Autodesk Inventor part; units mm, degrees
ref_plane "YZ Plane" through (0, 0, 0) normal (1, 0, 0) x (0, 1, 0)
ref_plane "XZ Plane" through (0, 0, 0) normal (0, 1, 0) x (-1, 0, 0)
ref_plane "XY Plane" through (0, 0, 0) normal (0, 0, 1) x (1, 0, 0)
sketch "Sketch1" plane through (0, 0, 0) normal (0, 1, 0) x (-1, 0, 0)
  circle A0 centre (0, 0) radius 3.5
  circle A1 centre (0, 0) radius 3.9
  circle A2 centre (0, 0) radius 0.5
  line L0 (3.9, 0) -> (3.9, 3.9)
  line L1 (3.9, 3.9) -> (0, 3.9)
  line L2 (-3.9, 0) -> (-3.9, 3.9)
  line L3 (-3.9, 3.9) -> (0, 3.9)
  line L4 (3.9, 3.9) -> (3.9, 5.9)
  line L5 (3.9, 5.9) -> (-3.9, 5.9)
  line L6 (-3.9, 5.9) -> (-3.9, 3.9)
  line L7 (3.9, 5.9) -> (10, 5.9)
  line L8 (10, 5.9) -> (10, 3.9)
  line L9 (10, 3.9) -> (3.9, 3.9)
  line L10 (-3.9, 5.9) -> (-10, 5.9)
  line L11 (-10, 5.9) -> (-10, 3.9)
  line L12 (-10, 3.9) -> (-3.9, 3.9)
  dimension "d0" = 7
  dimension "d1" = 7.8
  dimension "d2" = 1
  dimension "d7" = 2
  dimension "d10" = 20
extrude "Extrusion1" add sketch "Sketch1" along normal blind 8 contours A1 | A1 L1 L0 | L3 L6 L5 L4 L1 | A1 L2 L3 | L4 L7 L8 L9 | L12 L11 L10 L6
extrude "Extrusion2" add sketch "Sketch1" against normal blind 2 contours A0 | A1 | A1 L1 L0 | L3 L6 L5 L4 L1 | A1 L2 L3 | L4 L7 L8 L9 | L12 L11 L10 L6
sketch "Sketch2" plane through (10, 8, 3.9) normal (0, 0, -1) x (-1, 0, 0)
  circle A0 centre (3, -5) radius 1.5
  circle A1 centre (17, -5) radius 1.5
  line L0 (3, -5) -> (17, -5) construction
  line L1 (0, -10) -> (0, 0) construction
  line L2 (20, -10) -> (20, 0) construction
  line L3 (0, 0) -> (6.1, 0)
  line L4 (3, -3.5) -> (3, -3) construction
  line L5 (3, -3) -> (3.9922, -3.875)
  line L6 (3, -3) -> (2.0078, -3.875)
  line L7 (17, -3.5) -> (17, -3) construction
  line L8 (17, -3) -> (16.0078, -3.875)
  line L9 (17, -3) -> (17.9922, -3.875)
  point P0 (10, -8)
  dimension "d11" = 3
  dimension "d12" = 3
  dimension "d13" = 3
  dimension "d14" = 3
  dimension "d15" = 5
  dimension "d18" = 0.5
  dimension "d19" = 0.5
extrude "Extrusion3" cut sketch "Sketch2" against normal through all
equation "\"d13\" = d12"
equation "\"d14\" = d11"
equation "\"d19\" = d18"
properties part number "w_3DPrint"
Here's how the part is built. I have some questions about the finished solid (model axes, mm). A direction names the side the tool comes from. Give positions to 0.01 mm unless a question says otherwise; leave off trailing zeros. Order: outer loops, then holes, each group sorted by start corner. A loop starts at its lowest first (then second) coordinate and runs counter-clockwise, first axis right, second up. Notation, with made-up numbers: (39.5, -20.5) -> (78.5, -20.5) arc R32 ccw to (78.5, 5.5) -> close; hole circle Ø10 at (79, -30.5). An arc over 180 degrees is marked (long way). Use a Markdown table: item, result. Add a question column.
Item 1: Will these pins go through, and if not, where does the flat tip stop? pin 1 (1.2 mm diameter, centred on y = 2.5, z = 2, fed in from -X); pin 2 (2 mm diameter, centred on x = 6, y = 5.5, fed in from -Z); pin 3 (3.5 mm diameter, centred on x = 0.5, z = 1, fed in from +Y).
Item 2: Imagine slicing it at A-A on y = 3. Please give me the cut outline in (x, z).
Item 3: I need wall thicknesses on line 1 (X direction, y = 3, z = 4.95); line 2 (Z direction, x = 0, y = -0.85); line 3 (Z direction, x = -5, y = 7.5). Which ranges of each line are inside material? Lowest first, please.
Item 4: For faces 1 (the face through (-8.3, 1.8, 3.9)), 2 (the face through (3.9, 3, 2)), 3 (the face through (-3.233, 3.944, 1.341)), 4 (the face through (-7.49, 4.57, 4.89)), which set-ups out of +Z, -Z, +X, -X, +Y, -Y let a thin tool reach every point of the face, with its end or its side?
Item 5: If we mould it in two halves opening along Y, with no side actions, what happens to faces 5 (the face through (0, 0, -1)), 6 (the face through (7.49, 4.57, 4.89)), 7 (the face through (10, 3, 5))? For each: pulls with the +Y half, pulls with the -Y half, needs draft (parallel to the pull), parting line crosses it, or undercut.
Item 6: Imagine slicing it at D-D on z = -1. Please give me the cut outline in (x, y), plus the area to 3 significant figures.
Item 7: Imagine slicing it at B-B on x = 6.5. Please give me the cut outline in (y, z).
Item 8: Imagine slicing it at C-C on y = -0.75. Please give me the cut outline in (x, z).
Data:
| question | item | result |
|---|---|---|
| 1 | pin 1 | stops at x = -3.9 |
| 1 | pin 2 | stops at z = 3.9 |
| 1 | pin 3 | stops at y = 0 |
| 2 | outline | (-10, 3.9) -> (-8.5, 3.9) -> (-8.5, 5.9) -> (-10, 5.9) -> close; (-5.5, 3.9) -> (-3.9, 3.9) -> (-3.9, 0) arc R3.9 ccw to (3.9, 0) -> (3.9, 3.9) -> (5.5, 3.9) -> (5.5, 5.9) -> (-5.5, 5.9) -> close; (8.5, 3.9) -> (10, 3.9) -> (10, 5.9) -> (8.5, 5.9) -> close; hole circle Ø7 at (0, 0) |
| 3 | line 1 | x = -10 to -8.5, -5.5 to 5.5, 8.5 to 10 |
| 3 | line 2 | z = -3.9 to -0.5, 0.5 to 5.9 |
| 3 | line 3 | z = 3.9 to 5.9 |
| 4 | face 1 | -Z, -X, +Y, -Y |
| 4 | face 2 | -Z, +X, +Y, -Y |
| 4 | face 3 | +Y |
| 4 | face 4 | +Z, -Z |
| 5 | face 5 | pulls with the +Y half |
| 5 | face 6 | undercut |
| 5 | face 7 | needs draft |
| 6 | outline | (-3.77, -2) -> (3.77, -2) -> (3.77, 8) -> (3.35, 8) -> (3.35, 0) -> (-3.35, 0) -> (-3.35, 8) -> (-3.77, 8) -> close |
| 6 | area | 21.7 mm² |
| 7 | outline | (-2, 3.9) -> (1.59, 3.9) -> (1.59, 5.9) -> (-2, 5.9) -> close; (4.56, 3.9) -> (8, 3.9) -> (8, 5.9) -> (4.56, 5.9) -> close |
| 8 | outline | (-10, 3.9) -> (-3.9, 3.9) -> (-3.9, 0) arc R3.9 ccw to (3.9, 0) -> (3.9, 3.9) -> (10, 3.9) -> (10, 5.9) -> (-10, 5.9) -> close; hole circle Ø1 at (0, 0) |
